```python
from build123d import *

# Parameters (mm, degrees)
SCHIZZO1_W                   = 20.2
SCHIZZO1_H                   = 20.2
ESTRUSIONE_ESTRUSIONE1_DEPTH = 46
RACCORDO1_R                  = 20
SCHIZZO8_R                   = 2.5
TAGLIO_ESTRUSIONE3_DEPTH     = 5
TAGLIO_ESTRUSIONE4_DEPTH     = 106.540709324
RACCORDO2_R                  = 10
RACCORDO3_R                  = 4
SCHIZZO11_R                  = 2.5
TAGLIO_ESTRUSIONE5_DEPTH     = 106.540709324
ESTRUSIONE_ESTRUSIONE2_DEPTH = 46
RACCORDO4_R                  = 3
SCHIZZO11_3_R                = 2.5
TAGLIO_ESTRUSIONE6_DEPTH     = 106.540709324


with BuildPart() as part:
    # Schizzo1 → Estrusione-Estrusione1 (new body)
    with BuildSketch(Plane.XY):
        Polygon((25, 0), (-25, 0), (-35.161364738, 17.6), (-17.840856662, 27.6), (-47.840856662, 79.561524227), (-43.510729643, 82.061524227), (-13.510729643, 30.1), (13.510729643, 30.1), (43.510729643, 82.061524227), (47.840856662, 79.561524227), (17.840856662, 27.6), (35.161364738, 17.6), align=None)
        with Locations((0, 15)):
            Rectangle(SCHIZZO1_W, SCHIZZO1_H, mode=Mode.SUBTRACT)
    extrude(amount=ESTRUSIONE_ESTRUSIONE1_DEPTH)

    # Raccordo1
    raccordo1_edges = [part.edges().sort_by_distance(p)[0] for p in [
        (25, 0, 23),
        (-25, 0, 23),
    ]]
    fillet(raccordo1_edges, radius=RACCORDO1_R)

    # Schizzo8 → Taglio-Estrusione3 (cut)
    with BuildSketch(Plane(origin=(-1.429491924, -0.825317547, 0), x_dir=(0, 0, 1), z_dir=(-0.8660254037844398, -0.49999999999999806, 0))):
        with Locations(Location((10, 82.822729475, 0), (0, 0, 270))):
            Circle(SCHIZZO8_R)
        with Locations(Location((10, 47.822729475, 0), (0, 0, 270))):
            Circle(SCHIZZO8_R)
        with Locations(Location((36, 47.822729475, 0), (0, 0, 90))):
            Circle(SCHIZZO8_R)
        with Locations(Location((36, 82.822729475, 0), (0, 0, 270))):
            Circle(SCHIZZO8_R)
    taglio_estrusione3 = extrude(amount=-TAGLIO_ESTRUSIONE3_DEPTH, mode=Mode.SUBTRACT)

    # Specchia1: Taglio-Estrusione3 across plane
    add(taglio_estrusione3.mirror(Plane(origin=(0, 0, 0), x_dir=(0, 0, 1), z_dir=(1, 0, 0))), mode=Mode.SUBTRACT)

    # Schizzo10 → Taglio-Estrusione4 (cut, through all)
    with BuildSketch(Plane(origin=(0, 0, 0), x_dir=(-1, 0, 0), z_dir=(0, 0, -1))):
        with BuildLine():
            Line((-28.831237719, 16.635898385), (-13.452994616, 25.51453118))
            Line((-13.452994616, 25.51453118), (-13.452994616, 5))
            ThreePointArc((-13.452994616, 5), (-20.952994616, 7.009618943), (-26.443375673, 12.5))
            Line((-26.443375673, 12.5), (-28.831237719, 16.635898385))
        make_face()
        with BuildLine():
            Line((13.452994616, 25.51453118), (13.452994616, 5))
            ThreePointArc((13.452994616, 5), (20.952994616, 7.009618943), (26.443375673, 12.5))
            Line((26.443375673, 12.5), (28.831237719, 16.635898385))
            Line((28.831237719, 16.635898385), (13.452994616, 25.51453118))
        make_face()
    extrude(amount=-TAGLIO_ESTRUSIONE4_DEPTH, mode=Mode.SUBTRACT)

    # Raccordo2
    raccordo2_edges = [part.edges().sort_by_distance(p)[0] for p in [
        (-13.510729643, 30.1, 23),
        (13.510729643, 30.1, 23),
    ]]
    fillet(raccordo2_edges, radius=RACCORDO2_R)

    # Raccordo3
    raccordo3_edges = [part.edges().sort_by_distance(p)[0] for p in [
        (28.831237719, 16.635898385, 23),
        (13.452994616, 25.51453118, 23),
        (13.452994616, 5, 23),
        (-13.452994616, 5, 23),
        (-13.452994616, 25.51453118, 23),
        (-28.831237719, 16.635898385, 23),
    ]]
    fillet(raccordo3_edges, radius=RACCORDO3_R)

    # Schizzo11 → Taglio-Estrusione5 (cut, through all)
    with BuildSketch(Plane.XZ):
        with Locations((0, 35)):
            Circle(SCHIZZO11_R)
        with Locations((0, 11)):
            Circle(SCHIZZO11_R)
    extrude(amount=-TAGLIO_ESTRUSIONE5_DEPTH, mode=Mode.SUBTRACT)

    # Schizzo13 → Estrusione-Estrusione2 (add)
    with BuildSketch(Plane(origin=(0, 0, 0), x_dir=(-1, 0, 0), z_dir=(0, 0, -1))):
        Polygon((-33.717989065, 65.1), (33.717989065, 65.1), (30.831237719, 60.1), (-30.831237719, 60.1), align=None)
    extrude(amount=-ESTRUSIONE_ESTRUSIONE2_DEPTH)

    # Raccordo4
    raccordo4_edges = [part.edges().sort_by_distance(p)[0] for p in [
        (30.831237719, 60.1, 23),
        (33.717989065, 65.1, 23),
        (-33.717989065, 65.1, 23),
        (-30.831237719, 60.1, 23),
    ]]
    fillet(raccordo4_edges, radius=RACCORDO4_R)

    # Schizzo11<3> → Taglio-Estrusione6 (cut, through all)
    with BuildSketch(Plane.XZ):
        with Locations((0, 11)):
            Circle(SCHIZZO11_3_R)
    extrude(amount=-TAGLIO_ESTRUSIONE6_DEPTH, mode=Mode.SUBTRACT)


solid = part.part
```
The listing builds one solid part. Answer for the finished solid, in the listing's coordinates (mm). A direction names the side the tool comes from. Coordinates: 2 decimals unless noted, no trailing zeros. Write each loop counter-clockwise with the first axis right and the second up, starting at its lowest first coordinate (ties: lowest second). Pieces come first, ordered by that corner, then holes. Notation, with made-up numbers: (54, 66.25) - (102, 66.25) arc R15 cw to (102, 75.25) - close; hole circle Ø5 at (12.5, 51). An arc over 180 degrees is marked (long way). Return JSON: item names as keys, results as strings. Group by question number.
1. Straight lines are drawn through the part: L1, parallel to Z at x = 0, y = 3; L2, parallel to Y at x = -2, z = 32; L3, parallel to Y at x = -20, z = 23. For each, find the intervals that lie inside material, in ascending order.
2. Which of the six approach directions +Z, -Z, +X, -X, +Y, -Y give full straight-line access (tool end or side, diameter ignored) to faces 4 (the cylindrical face through (-0.54, 62.56, 8.56)), 5 (the flat face through (-32.631, 53.217, 22.678)), 6 (the cylindrical face through (-0.54, 27.56, 32.56)), 7 (the cylindrical face through (33.5, 65.51, 23.32)), 8 (the flat face through (10.1, 15, 23))?
3. A cutting plane is placed at A-A, the plane x = 0. Give the number of separate pieces and of enclosed holes in the cut face, plus the area to 3 significant figures.
4. A cutting plane is placed at B-B, the plane y = 59. Determine the outline of the cut face in (x, z).
5. Determine the mould class of faces 1 (the cylindrical face through (-15.4, 22.02, 23.32)), 2 (the cylindrical face through (-0.54, 27.56, 8.56)), 3 (the cylindrical face through (-33.5, 65.51, 23.32)) for opening direction Y: released by +Y, released by -Y, zero draft, split by the parting line, or undercut.
6. Given pin 1 (10 mm diameter, centred on x = -2, z = 31, fed in from +Y); pin 2 (1 mm diameter, centred on y = 47, z = 26.5, fed in from +X); pin 3 (6 mm diameter, centred on y = 9, z = 40, fed in from -X), each flat-ended and moving along its own axis, determine where each tip first touches the part or whether it passes through.
Ans:
{
 "1": {"L1": "0 to 8.5, 13.5 to 32.5, 37.5 to 46", "L2": "0 to 4.9, 25.1 to 30.1, 60.1 to 65.1", "L3": "1.1 to 6.5, 21.73 to 26.35, 31.34 to 41.34, 60.1 to 65.1"},
 "2": {"face 4": "+Y, -Y", "face 5": "+Z, -Z, -X", "face 6": "-Y", "face 7": "+Z, -Z, +Y", "face 8": "+Z, -Z"},
 "3": {"separate pieces": "8", "enclosed holes": "0", "area": "561 mm²"},
 "4": {"outline": "(-35.97, 0) - (-27.96, 0) - (-27.96, 46) - (-35.97, 46) - close; (27.96, 0) - (35.97, 0) - (35.97, 46) - (27.96, 46) - close"},
 "5": {"face 1": "undercut", "face 2": "zero draft", "face 3": "released by +Y"},
 "6": {"pin 1": "y = 65.1", "pin 2": "x = 29.33", "pin 3": "x = -31.93"}
}
